```python
from build123d import *

# Parameters (mm, degrees)
SKETCH1_W                     = 33.3
SKETCH1_H                     = 10.3
BOSS_EXTRUDE1_DEPTH           = 1.9
SKETCH2_W                     = 24.5
SKETCH2_H                     = 6.2
SKETCH2_R                     = 1.5
BOSS_EXTRUDE2_DEPTH           = 3
SKETCH3_W                     = 4.5
SKETCH3_H                     = 6.2
BOSS_EXTRUDE3_DEPTH           = 7.5
SKETCH4_W                     = 6
SKETCH4_H                     = 10.3
BOSS_EXTRUDE4_DEPTH           = 10
SKETCH5_R                     = 1
BOSS_EXTRUDE5_DEPTH           = 2
BOSS_EXTRUDE5_DRAFT           = 22
BOSS_EXTRUDE5_PROFILE_2_DEPTH = 2
BOSS_EXTRUDE5_PROFILE_2_DRAFT = 22
BOSS_EXTRUDE5_PROFILE_3_DEPTH = 2
BOSS_EXTRUDE5_PROFILE_3_DRAFT = 22
BOSS_EXTRUDE5_PROFILE_4_DEPTH = 2
BOSS_EXTRUDE5_PROFILE_4_DRAFT = 22
SKETCH6_W                     = 4
SKETCH6_H                     = 1
CUT_EXTRUDE1_DEPTH            = 4.5
CUT_EXTRUDE2_REACH            = 23.103
SKETCH2_2_R                   = 1.5


with BuildPart() as part:
    # Sketch1 → Boss-Extrude1 (new body)
    with BuildSketch(Plane(origin=(0, 0, 0), x_dir=(1, 0, 0), z_dir=(0, 1, 0))):
        Rectangle(SKETCH1_W, SKETCH1_H)
    extrude(amount=BOSS_EXTRUDE1_DEPTH)

    # Sketch2 → Boss-Extrude2 (add)
    with BuildSketch(Plane(origin=(0, 1.9, 0), x_dir=(1, 0, 0), z_dir=(0, 1, 0))):
        with Locations((3.8, 0)):
            Rectangle(SKETCH2_W, SKETCH2_H)
        with Locations(Location((-5.95, 0, 0), (0, 0, 270))):
            Circle(SKETCH2_R, mode=Mode.SUBTRACT)
        with Locations(Location((13.55, 0, 0), (0, 0, 270))):
            Circle(SKETCH2_R, mode=Mode.SUBTRACT)
    extrude(amount=BOSS_EXTRUDE2_DEPTH)

    # Sketch3 → Boss-Extrude3 (add)
    with BuildSketch(Plane(origin=(0, 4.9, 0), x_dir=(1, 0, 0), z_dir=(0, 1, 0))):
        with Locations((0.05, 0)):
            Rectangle(SKETCH3_W, SKETCH3_H)
        with Locations((7.55, 0)):
            Rectangle(SKETCH3_W, SKETCH3_H)
    extrude(amount=BOSS_EXTRUDE3_DEPTH)

    # Sketch4 → Boss-Extrude4 (add)
    with BuildSketch(Plane.XZ):
        with Locations((-13.65, 0)):
            Rectangle(SKETCH4_W, SKETCH4_H)
    extrude(amount=BOSS_EXTRUDE4_DEPTH)


with BuildPart() as boss_extrude5_tool:
    # Sketch5 → Boss-Extrude5 (with draft: the straight prism first)
    with BuildSketch(Plane.XZ):
        with Locations((-0.925, 1.726795989)):
            Circle(SKETCH5_R)
    extrude(amount=BOSS_EXTRUDE5_DEPTH)
    # Boss-Extrude5: the draft: its side faces are tilted about the plane it starts from
    boss_extrude5_sides = [boss_extrude5_tool.faces().sort_by_distance(p)[0] for p in [
        (-1.925, -1, 1.726795989),
    ]]
    draft(boss_extrude5_sides, Plane.XZ, BOSS_EXTRUDE5_DRAFT)


with BuildPart() as part_1:
    add(part.part)

    # Boss-Extrude5: add boss_extrude5_tool
    add(boss_extrude5_tool.part)


with BuildPart() as boss_extrude5_profile_2_tool:
    # Sketch5 → Boss-Extrude5 profile 2 (with draft: the straight prism first)
    with BuildSketch(Plane.XZ):
        with Locations((-0.925, -0.973204011)):
            Circle(SKETCH5_R)
    extrude(amount=BOSS_EXTRUDE5_PROFILE_2_DEPTH)
    # Boss-Extrude5 profile 2: the draft: its side faces are tilted about the plane it starts from
    boss_extrude5_profile_2_sides = [boss_extrude5_profile_2_tool.faces().sort_by_distance(p)[0] for p in [
        (-1.925, -1, -0.973204011),
    ]]
    draft(boss_extrude5_profile_2_sides, Plane.XZ, BOSS_EXTRUDE5_PROFILE_2_DRAFT)


with BuildPart() as part_2:
    add(part_1.part)

    # Boss-Extrude5 profile 2: add boss_extrude5_profile_2_tool
    add(boss_extrude5_profile_2_tool.part)


with BuildPart() as boss_extrude5_profile_3_tool:
    # Sketch5 → Boss-Extrude5 profile 3 (with draft: the straight prism first)
    with BuildSketch(Plane.XZ):
        with Locations((8.525, -0.973204011)):
            Circle(SKETCH5_R)
    extrude(amount=BOSS_EXTRUDE5_PROFILE_3_DEPTH)
    # Boss-Extrude5 profile 3: the draft: its side faces are tilted about the plane it starts from
    boss_extrude5_profile_3_sides = [boss_extrude5_profile_3_tool.faces().sort_by_distance(p)[0] for p in [
        (7.525, -1, -0.973204011),
    ]]
    draft(boss_extrude5_profile_3_sides, Plane.XZ, BOSS_EXTRUDE5_PROFILE_3_DRAFT)


with BuildPart() as part_3:
    add(part_2.part)

    # Boss-Extrude5 profile 3: add boss_extrude5_profile_3_tool
    add(boss_extrude5_profile_3_tool.part)


with BuildPart() as boss_extrude5_profile_4_tool:
    # Sketch5 → Boss-Extrude5 profile 4 (with draft: the straight prism first)
    with BuildSketch(Plane.XZ):
        with Locations((8.525, 1.726795989)):
            Circle(SKETCH5_R)
    extrude(amount=BOSS_EXTRUDE5_PROFILE_4_DEPTH)
    # Boss-Extrude5 profile 4: the draft: its side faces are tilted about the plane it starts from
    boss_extrude5_profile_4_sides = [boss_extrude5_profile_4_tool.faces().sort_by_distance(p)[0] for p in [
        (7.525, -1, 1.726795989),
    ]]
    draft(boss_extrude5_profile_4_sides, Plane.XZ, BOSS_EXTRUDE5_PROFILE_4_DRAFT)


with BuildPart() as part_4:
    add(part_3.part)

    # Boss-Extrude5 profile 4: add boss_extrude5_profile_4_tool
    add(boss_extrude5_profile_4_tool.part)

    # Sketch6 → Cut-Extrude1 (cut)
    with BuildSketch(Plane(origin=(0, 12.4, 0), x_dir=(1, 0, 0), z_dir=(0, 1, 0))):
        with Locations((3.8, 0)):
            Rectangle(SKETCH6_W, SKETCH6_H)
    extrude(amount=-CUT_EXTRUDE1_DEPTH, mode=Mode.SUBTRACT)

    # Sketch2_2 → Cut-Extrude2 (cut, up to next)
    with BuildSketch(Plane(origin=(0, 1.9, 0), x_dir=(1, 0, 0), z_dir=(0, 1, 0)), mode=Mode.PRIVATE) as cut_extrude2_sk1:
        with Locations(Location((13.55, 0, 0), (0, 0, 90))):
            Circle(SKETCH2_2_R)
    cut_extrude2_tool1 = extrude(cut_extrude2_sk1.sketch, amount=-CUT_EXTRUDE2_REACH, mode=Mode.PRIVATE) & part_4.part
    # Sketch2_2 → Cut-Extrude2 (cut, up to next)
    with BuildSketch(Plane(origin=(0, 1.9, 0), x_dir=(1, 0, 0), z_dir=(0, 1, 0)), mode=Mode.PRIVATE) as cut_extrude2_sk2:
        with Locations(Location((-5.95, 0, 0), (0, 0, 90))):
            Circle(SKETCH2_2_R)
    cut_extrude2_tool2 = extrude(cut_extrude2_sk2.sketch, amount=-CUT_EXTRUDE2_REACH, mode=Mode.PRIVATE) & part_4.part
    add(cut_extrude2_tool1.solids().sort_by_distance((13.55, 1.9, 0))[0], mode=Mode.SUBTRACT)
    add(cut_extrude2_tool2.solids().sort_by_distance((-5.95, 1.9, 0))[0], mode=Mode.SUBTRACT)


solid = part_4.part
```
The listing builds one solid part. Answer for the finished solid, in the listing's coordinates (mm). A direction names the side the tool comes from. Give positions to 0.01 mm unless a question says otherwise; leave off trailing zeros. Order: outer loops, then holes, each group sorted by start corner. A loop starts at its lowest first (then second) coordinate and runs counter-clockwise, first axis right, second up. Notation, with made-up numbers: (85.25, 21) -> (107.25, 21) arc R31 cw to (107.25, 54) -> close; hole circle Ø6 at (25.5, -28). An arc over 180 degrees is marked (long way). Answer as CSV lines item,"result". Start each with the question number.
Q1. Which of the six approach directions +Z, -Z, +X, -X, +Y, -Y give full straight-line access (tool end or side, diameter ignored) to faces 4 (the flat face through (4, 4.9, 0)), 5 (the conical face through (8.014, -1.208, -0.951)), 6 (the flat face through (16.65, 1, 0)), 7 (the flat face through (12, 4.9, -1)), 8 (the flat face through (-8.45, 3, 0))?
Q2. Determine the mould class of faces 1 (the flat face through (16.05, 3, 0)), 2 (the flat face through (1.8, 10, 0)), 3 (the flat face through (3.6, 4.7, 3.1)) for opening direction X: pulls with the +X half, pulls with the -X half, needs draft (parallel to the pull), parting line crosses it, or undercut.
Q3. Find the intervals of material crossed by L1, parallel to X at y = 0.8, z = 0; L2, parallel to X at y = 3.65, z = 0; L3, parallel to Z at x = -5.95, y = 4.25, in increasing order.
Q4. A cutting plane is placed at C-C (x = 7). Determine the outline of the cut face in (y, z), then the cut area to 3 significant figures.
Q5. Given pin 1 (3 mm diameter, centred on x = 9, z = -1, fed in from -Y); pin 2 (1.1 mm diameter, centred on y = 11, z = 0, fed in from -X); pin 3 (0.6 mm diameter, centred on x = 2, z = 0, fed in from +Y); pin 4 (5 mm diameter, centred on y = 8, z = 1, fed in from +X), each flat-ended and moving along its own axis, determine where each tip first touches the part or whether it passes through.
Q6. A cutting plane is placed at D-D (z = 3.5). Determine the outline of the cut face in (x, y), then the cut area to 3 significant figures.
Q7. A cutting plane is placed at A-A (x = 13.55). Determine the outline of the cut face in (y, z), then the cut area to 3 significant figures.
Q8. A cutting plane is placed at B-B (y = 9.25). Determine the outline of the cut face in (x, z), then the cut area to 3 significant figures.
Results found:
1,face 4,"+Z, -Z, +Y"
1,face 5,"-Y"
1,face 6,"+Z, -Z, +X, +Y, -Y"
1,face 7,"+Z, -Z, +X, +Y"
1,face 8,"+Z, -Z, -X, +Y"
2,face 1,"pulls with the +X half"
2,face 2,"undercut"
2,face 3,"needs draft"
3,L1,"-16.65 to -7.45, -4.45 to 12.05, 15.05 to 16.65"
3,L2,"-8.45 to -7.45, -4.45 to 12.05, 15.05 to 16.05"
3,L3,"-3.1 to -1.5, 1.5 to 3.1"
4,outline,"(0, -5.15) -> (1.9, -5.15) -> (1.9, -3.1) -> (12.4, -3.1) -> (12.4, 3.1) -> (1.9, 3.1) -> (1.9, 5.15) -> (0, 5.15) -> close"
4,area,"84.7 mm2"
5,pin 1,"y = -2"
5,pin 2,"x = -2.2"
5,pin 3,"y = 12.4"
5,pin 4,"x = 9.8"
6,outline,"(-16.65, -10) -> (-10.65, -10) -> (-10.65, 0) -> (16.65, 0) -> (16.65, 1.9) -> (-16.65, 1.9) -> close"
6,area,"123 mm2"
7,outline,"(0, -5.15) -> (1.9, -5.15) -> (1.9, -3.1) -> (4.9, -3.1) -> (4.9, -1.5) -> (0, -1.5) -> close; (0, 1.5) -> (4.9, 1.5) -> (4.9, 3.1) -> (1.9, 3.1) -> (1.9, 5.15) -> (0, 5.15) -> close"
7,area,"23.5 mm2"
8,outline,"(-2.2, -3.1) -> (2.3, -3.1) -> (2.3, -0.5) -> (1.8, -0.5) -> (1.8, 0.5) -> (2.3, 0.5) -> (2.3, 3.1) -> (-2.2, 3.1) -> close; (5.3, -3.1) -> (9.8, -3.1) -> (9.8, 3.1) -> (5.3, 3.1) -> (5.3, 0.5) -> (5.8, 0.5) -> (5.8, -0.5) -> (5.3, -0.5) -> close"
8,area,"54.8 mm2"
